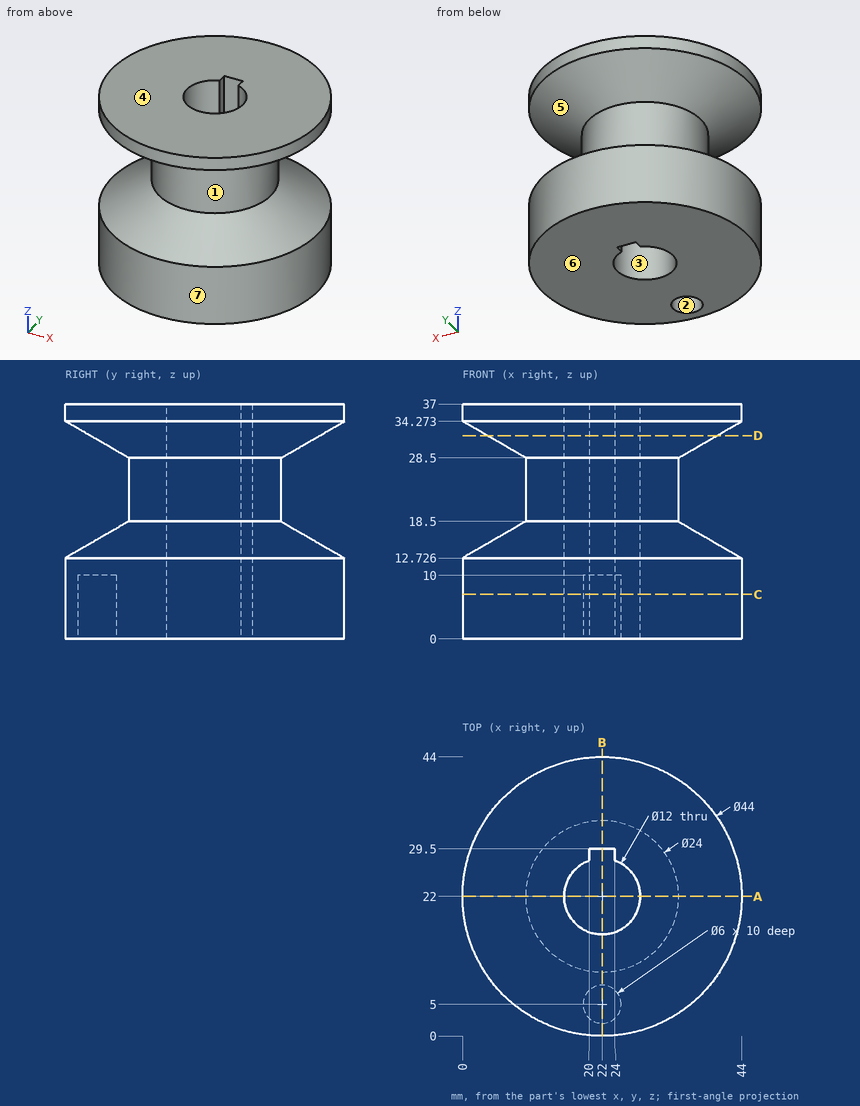
Can you work these out from the drawing? Everything is in mm from the part's minimum corner. A direction names the side the tool comes from. Give positions to 0.01 mm unless a question says otherwise; leave off trailing zeros. Order: outer loops, then holes, each group sorted by start corner. A loop starts at its lowest first (then second) coordinate and runs counter-clockwise, first axis right, second up. Notation, with made-up numbers: M 15,-2 L 35,-2 A30 cw 35,33 Z; hole C 24.25,-9 d8. An arc over 180 degrees is marked long. Use a Markdown table: item, result. Add a question column.
Item 1: Will these pins go through, and if not, where does the flat tip stop? pin 1 (4.5 mm diameter, centred on x = 22.5, z = 15.5, fed in from -Y) (1 decimal); pin 2 (2 mm diameter, centred on y = 28.5, z = 19.5, fed in from +X) (1 decimal); pin 3 (5 mm diameter, centred on y = 11.5, z = 24, fed in from +X) (1 decimal); pin 4 (3 mm diameter, centred on x = 23.5, y = 6.5, fed in from -Z).
Item 2: Suppose I cut it at B-B (x = 22). List the corners of the cut face in (y, z) for me, then the cut area to 3 significant figures.
Item 3: We'd pull the mould along Z, two halves only. Please class the marked faces 4, 5, 6 and 7: +Z half, -Z half, draft (parallel to the pull), parting line (faces both ways), or undercut.
Item 4: Suppose I cut it at A-A (y = 22). List the corners of the cut face in (x, z) for me.
Item 5: Suppose I cut it at C-C (z = 7). List the corners of the cut face in (x, y) for me, then the cut area to 3 significant figures.
Item 6: If I drill on L1, parallel to X at y = 22, z = 11; L2, parallel to X at y = 18.5, z = 30 (1 decimal); L3, parallel to Z at x = 5, y = 31.5 (1 decimal), over which ranges is the centre line in solid material (lowest first)? Write a range as [from, to].
Item 7: For the marked faces 1, 2 and 3, which set-ups out of +Z, -Z, +X, -X, +Y, -Y let a thin tool reach every point of the face, with its end or its side?
Item 8: Suppose I cut it at D-D (z = 32). List the corners of the cut face in (x, y) for me (1 decimal).
Answer sheet:
| question | item | result |
|---|---|---|
| 1 | pin 1 | stops at y = 0.9 |
| 1 | pin 2 | stops at x = 32.7 |
| 1 | pin 3 | stops at x = 30.9 |
| 1 | pin 4 | stops at z = 0 |
| 2 | outline | M 0,0 L 2,0 L 2,10 L 8,10 L 8,0 L 16,0 L 16,37 L 0,37 L 0,34.27 L 10,28.5 L 10,18.5 L 0,12.73 Z; M 29.5,0 L 44,0 L 44,12.73 L 34,18.5 L 34,28.5 L 44,34.27 L 44,37 L 29.5,37 Z |
| 2 | area | 753 mm² |
| 3 | face 4 | +Z half |
| 3 | face 5 | undercut |
| 3 | face 6 | -Z half |
| 3 | face 7 | draft |
| 4 | outline | M 0,0 L 16,0 L 16,37 L 0,37 L 0,34.27 L 10,28.5 L 10,18.5 L 0,12.73 Z; M 28,0 L 44,0 L 44,12.73 L 34,18.5 L 34,28.5 L 44,34.27 L 44,37 L 28,37 Z |
| 5 | outline | C 22,22 d44; hole C 22,5 d6; hole M 20,27.66 A6 ccw long 24,27.66 L 24,29.5 L 20,29.5 Z |
| 5 | area | 1,370 mm² |
| 6 | L1 | x = [0, 16], [28, 44] |
| 6 | L2 | x = [7.8, 17.1], [26.9, 36.2] |
| 6 | L3 | z = [0, 14.2], [32.8, 37] |
| 7 | face 1 | none |
| 7 | face 2 | -Z |
| 7 | face 3 | +Z, -Z |
| 8 | outline | C 22,22 d36.1; hole M 20,27.7 A6 ccw long 24,27.7 L 24,29.5 L 20,29.5 Z |
